Design review of the part shown in the three views and the two pictorial views. Dimensions are in mm from the part's minimum x, y and z. A direction names the side the tool comes from. Give positions to 0.01 mm unless a question says otherwise; leave off trailing zeros. Loops run counter-clockwise (first coordinate to the right, second up) from the corner with the lowest first, then second, coordinate; pieces in that order, holes last.
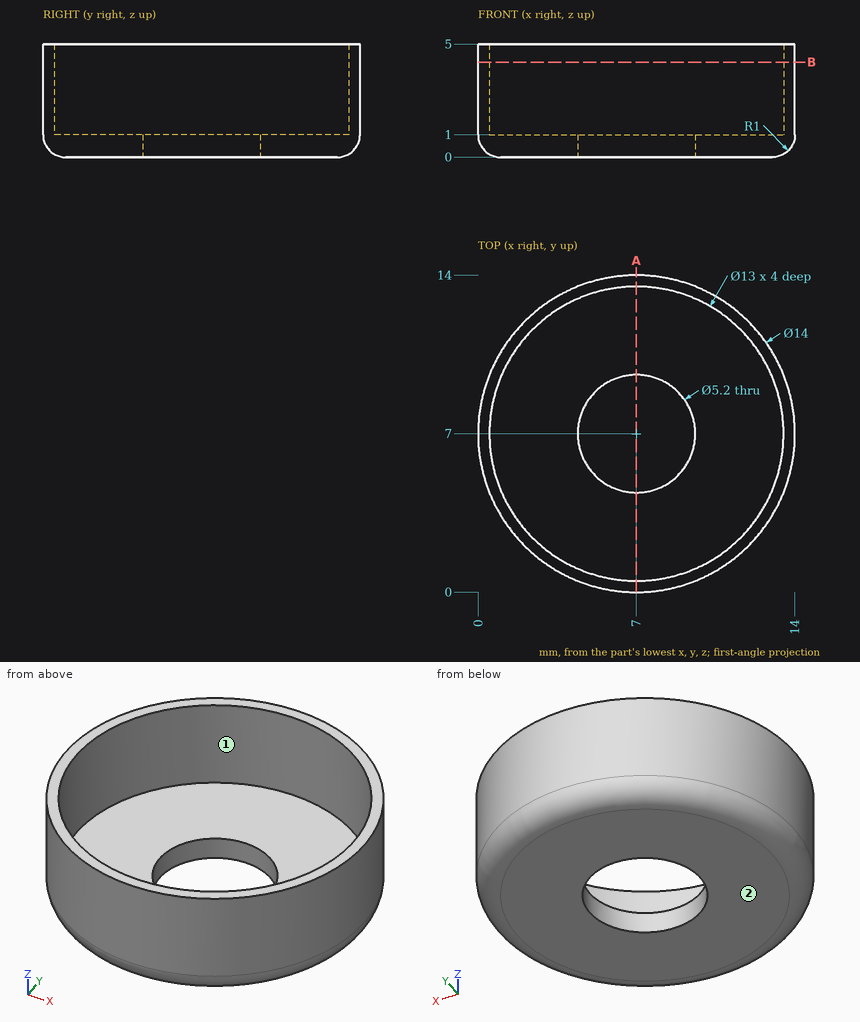
Q1. Wall thickness on line 1 (Y direction, x = 7, z = 2.9); line 2 (Z direction, x = 11, y = 8.5); line 3 (Y direction, x = 12.75, z = 4.8): over which ranges is each line inside the solid? List them lowest first.
Results:
line 1: y = 0 to 0.5, 13.5 to 14
line 2: z = 0 to 1
line 3: y = 3.01 to 3.97, 10.03 to 10.99
Q2. Insertion check: pin 1 (2 mm diameter, centred on x = 11, y = 5, fed in from +Z); pin 2 (1.5 mm diameter, centred on x = 3, y = 4, fed in from -Z); pin 3 (1.5 mm diameter, centred on x = 6, z = 2, fed in from -Y); pin 4 (1.5 mm diameter, centred on x = 12.5, z = 3, fed in from +Y). Each pin has a flat end and moves straight along its axis. Give the tip position at first contact, or say it passes through.
Results:
pin 1: stops at z = 1
pin 2: stops at z = 0
pin 3: stops at y = 0
pin 4: stops at y = 12.14
Q3. Tool access review of the marked faces 1 and 2: name each direction out of +Z, -Z, +X, -X, +Y, -Y from which nothing blocks a thin tool from reaching the whole face with its end or side.
Results:
face 1: +Z
face 2: -Z, +X, -X, +Y, -Y
Q4. Take a section at B-B (z = 4.2). Give the boundary of the cut face in (x, y).
Results:
outline: circle Ø14 at (7, 7); hole circle Ø13 at (7, 7)
Q5. Take a section at A-A (x = 7). Give the boundary of the cut face in (y, z).
Results:
outline: (0, 1) arc R1 ccw to (1, 0) - (4.4, 0) - (4.4, 1) - (0.5, 1) - (0.5, 5) - (0, 5) - close; (9.6, 0) - (13, 0) arc R1 ccw to (14, 1) - (14, 5) - (13.5, 5) - (13.5, 1) - (9.6, 1) - close
